Input: dimensioned drawing with shaded views. Units: mm. Origin: part minimum x, y, z. A direction names the side the tool comes from. Give positions to 0.01 mm unless a question says otherwise; leave off trailing zeros. Order: outer loops, then holes, each group sorted by start corner. A loop starts at its lowest first (then second) coordinate and runs counter-clockwise, first axis right, second up. Notation, with made-up numbers: M 26,48.25 L 47,48.25 A17 cw 47,80.25 Z; hole C 14.25,36.5 d7. An arc over 180 degrees is marked long. Answer in a Markdown table with one row per item. Add a question column.
(1) Section query D-D, the plane y = 31. Return loops of the section in (x, z).
(2) Set-up query: the marked faces 1, 2 and 3. Return all of +Z, -Z, +X, -X, +Y, -Y with unobstructed straight access to the full face (end or side cutting, diameter ignored); none if empty.
(3) Pin query (flat end, axial travel): P1, Ø20, axis at x = 20, y = 65, coming from the -Z side; P2, Ø3, axis at y = 35.5, z = 34, coming from the +X side; P3, Ø1.5, axis at x = 30.5, z = 50, coming from the -Y side. Return the tip coordinate at first contact, or that it passes through.
(4) Material intervals for line 1 along Z through (x, y) = (41, 32); line 2 along Z through (x, y) = (37.5, 49); line 3 along X through (y, z) = (37, 14.5), sorted ascending.
(5) Section query B-B, the plane x = 7. Return loops of the section in (y, z).
(6) Section query A-A, the plane x = 13. Return loops of the section in (y, z), plus the area to 3 significant figures.
(7) Section query C-C, the plane z = 34. Return loops of the section in (x, y).
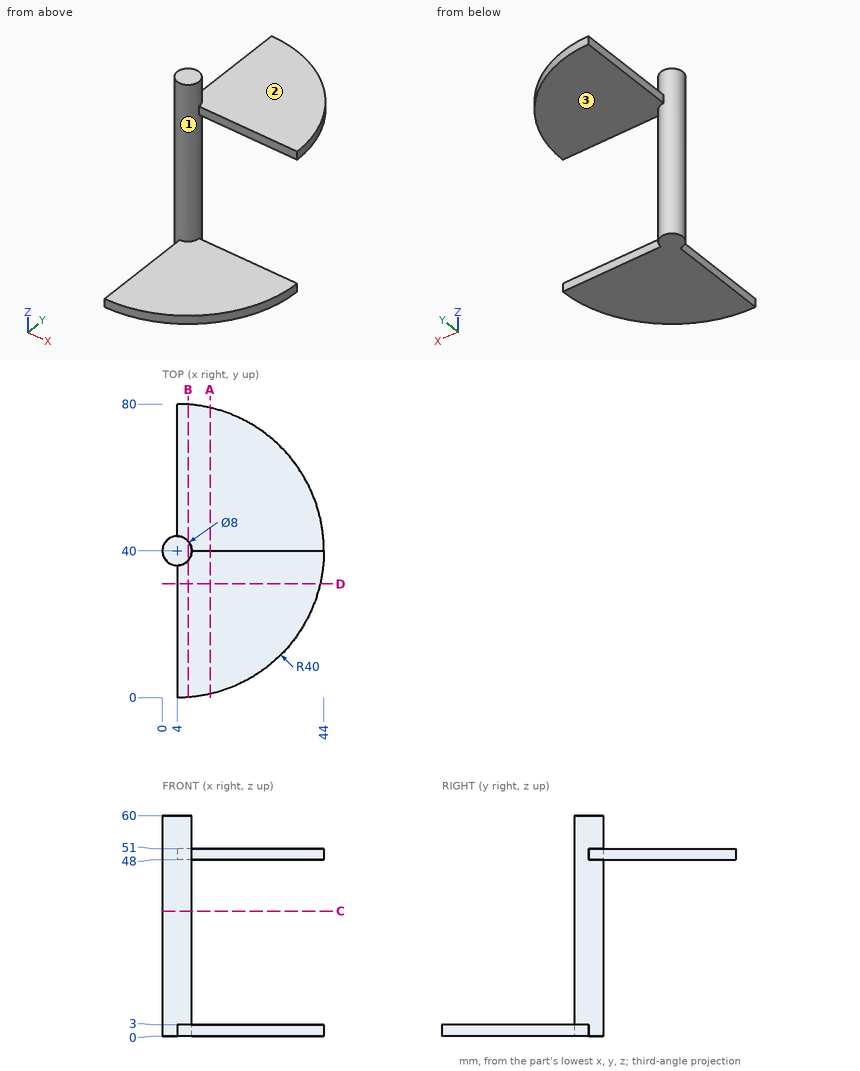
Values follow:
| question | item | result |
|---|---|---|
| 1 | outline | M 4,0 L 42.97,0 L 42.97,3 L 4,3 Z |
| 2 | face 1 | none |
| 2 | face 2 | +Z, +X, +Y |
| 2 | face 3 | -Z, +X, +Y |
| 3 | P1 | stops at z = 48 |
| 3 | P2 | stops at x = 6.65 |
| 3 | P3 | stops at y = 40 |
| 4 | line 1 | z = 0 to 3 |
| 4 | line 2 | z = 48 to 51 |
| 4 | line 3 | x = 1.35 to 6.65 |
| 5 | outline | M 0.11,0 L 42.65,0 L 42.65,48 L 79.89,48 L 79.89,51 L 42.65,51 L 42.65,60 L 37.35,60 L 37.35,3 L 0.11,3 Z |
| 6 | outline | M 1.03,0 L 40,0 L 40,3 L 1.03,3 Z; M 40,48 L 78.97,48 L 78.97,51 L 40,51 Z |
| 6 | area | 234 mm² |
| 7 | outline | C 4,40 d8 |
